Geometry check sheet. Reference: the model listing, model coordinates, mm. Give positions to 0.01 mm unless a question says otherwise; leave off trailing zeros. Order: outer loops, then holes, each group sorted by start corner. A loop starts at its lowest first (then second) coordinate and runs counter-clockwise, first axis right, second up. Notation, with made-up numbers: (40.25, -31) - (96.25, -31) arc R29 cw to (96.25, 5) - close; hole circle Ø7 at (30.5, 24.5). An arc over 180 degrees is marked (long way). Put each result on its own line as item: value. Start each with the question number.
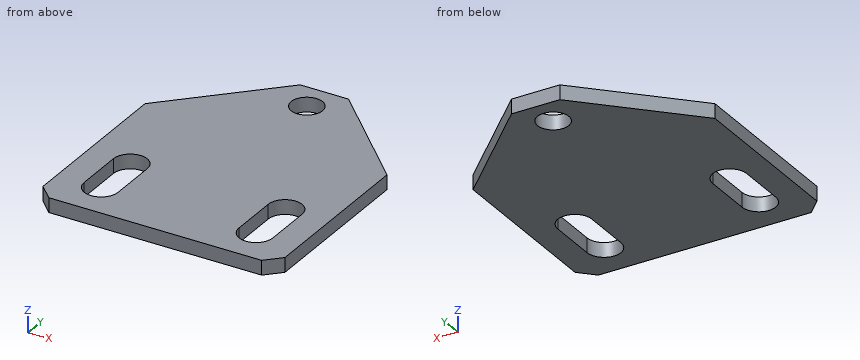
```python
from build123d import *

# Parameters (mm, degrees)
SKETCH_1_W             = 50
SKETCH_1_H             = 58
SM_BASE_FLANGE_1_DEPTH = 3
SKETCH_2_R             = 3.25
CUT_EXTRUDE_1_DEPTH    = 10
HOLE_WIZARD_7_0_7_1_D  = 7
CHAMFER_1_SIZE         = 3
CUT_EXTRUDE_2_DEPTH    = 10
CUT_EXTRUDE_3_DEPTH    = 10


# Sheet-metal steps are written as plain solids
with BuildPart() as part:
    # Sketch 1 → 基体-法兰1 (new body)
    with BuildSketch(Plane.XY):
        Rectangle(SKETCH_1_W, SKETCH_1_H)
    extrude(amount=-SM_BASE_FLANGE_1_DEPTH)

    # Sketch 2 → 切除-拉伸1 (cut)
    with BuildSketch(Plane.XY):
        with Locations((0, 23)):
            Circle(SKETCH_2_R)
    extrude(amount=-CUT_EXTRUDE_1_DEPTH, mode=Mode.SUBTRACT)

    # Ø7.0 (7) 直径孔1 (through all)
    with Locations(Plane.XY):
        with Locations((-16, -11.5), (16, -11.5)):
            Hole(HOLE_WIZARD_7_0_7_1_D / 2)

    # 倒角1
    chamfer_1_edges = [part.edges().sort_by_distance(p)[0] for p in [
        (25, -29, -1.5),
        (-25, -29, -1.5),
    ]]
    chamfer(chamfer_1_edges, length=CHAMFER_1_SIZE)

    # 草图5 → 切除-拉伸2 (cut)
    with BuildSketch(Plane.XY):
        Polygon((-5, 29), (-25, 9), (-25, 29), align=None)
        Polygon((25, 29), (5, 29), (25, 9), align=None)
    extrude(amount=-CUT_EXTRUDE_2_DEPTH, mode=Mode.SUBTRACT)

    # 草图7 → 切除-拉伸3 (cut)
    with BuildSketch(Plane.XY):
        with BuildLine():
            Line((-19.5, -21), (-19.5, -11))
            ThreePointArc((-19.5, -11), (-16, -7.5), (-12.5, -11))
            Line((-12.5, -11), (-12.5, -21))
            ThreePointArc((-12.5, -21), (-16, -24.5), (-19.5, -21))
        make_face()
        with BuildLine():
            Line((12.5, -21), (12.5, -11))
            ThreePointArc((12.5, -11), (16, -7.5), (19.5, -11))
            Line((19.5, -11), (19.5, -21))
            ThreePointArc((19.5, -21), (16, -24.5), (12.5, -21))
        make_face()
    extrude(amount=-CUT_EXTRUDE_3_DEPTH, mode=Mode.SUBTRACT)


solid = part.part
```
Item 1: Gauge pin test, flat ends, axial feed: pin 1 Ø10 at (x, y) = (-16, -8.5) entering from -Z; pin 2 Ø1.5 at (x, z) = (-13, -2.5) entering from +Y. Record the tip position at first contact, or that the pin passes through.
Item 2: Cross-section at B-B (z = -1.15). Enter the section's corners in (x, y), and give its area (3 significant figures).
Item 3: Cross-section at D-D (x = 16). Enter the section's corners in (y, z).
Item 4: Cross-section at C-C (y = -17). Enter the section's corners in (x, z), and give its area (3 significant figures).
Item 5: Cross-section at A-A (y = 23). Enter the section's corners in (x, z), and give its area (3 significant figures).
Item 6: Thickness scan on line 1 along X through (y, z) = (-20, -1.1); line 2 along Y through (x, z) = (0, -1.5); line 3 along X through (y, z) = (-22, -0.5). Record the ranges inside material, lowest first.
Recorded:
1. pin 1: stops at z = -3
1. pin 2: stops at y = 21.75
2. outline: (-25, -26) - (-22, -29) - (22, -29) - (25, -26) - (25, 9) - (5, 29) - (-5, 29) - (-25, 9) - close; hole (-19.5, -21) arc R3.5 ccw to (-12.5, -21) - (-12.5, -11) arc R3.5 ccw to (-19.5, -11) - close; hole circle Ø6.5 at (0, 23); hole (12.5, -21) arc R3.5 ccw to (19.5, -21) - (19.5, -11) arc R3.5 ccw to (12.5, -11) - close
2. area: 2,240 mm^2
3. outline: (-29, -3) - (-24.5, -3) - (-24.5, 0) - (-29, 0) - close; (-7.5, -3) - (18, -3) - (18, 0) - (-7.5, 0) - close
4. outline: (-25, -3) - (-19.5, -3) - (-19.5, 0) - (-25, 0) - close; (-12.5, -3) - (12.5, -3) - (12.5, 0) - (-12.5, 0) - close; (19.5, -3) - (25, -3) - (25, 0) - (19.5, 0) - close
4. area: 108 mm^2
5. outline: (-11, -3) - (-3.25, -3) - (-3.25, 0) - (-11, 0) - close; (3.25, -3) - (11, -3) - (11, 0) - (3.25, 0) - close
5. area: 46.5 mm^2
6. line 1: x = -25 to -19.5, -12.5 to 12.5, 19.5 to 25
6. line 2: y = -29 to 19.75, 26.25 to 29
6. line 3: x = -25 to -19.35, -12.65 to 12.65, 19.35 to 25
